Model file for the job. Use its own axes, mm. A direction names the side the tool comes from. Round coordinates to 2 decimals unless told otherwise and drop trailing zeros. Order: outer loops, then holes, each group sorted by start corner. A loop starts at its lowest first (then second) coordinate and runs counter-clockwise, first axis right, second up. Notation, with made-up numbers: (11.25, -25.75) - (68.25, -25.75) arc R18 cw to (68.25, -7.75) - close; hole circle Ø11 at (-5, 11.25). An arc over 180 degrees is marked (long way). Write item = value, one per line.
```python
from build123d import *

# Parameters (mm, degrees)
SKETCH_1_W          = 40
SKETCH_1_H          = 270
EXTRUDE_1_DEPTH     = 17
CUT_EXTRUDE_1_DEPTH = 6


with BuildPart() as part:
    # 스케치1 → 보스-돌출1 (new, symmetric)
    with BuildSketch(Plane(origin=(0, 0, 0), x_dir=(0, 0, -1), z_dir=(1, 0, 0))):
        with Locations((0, -135)):
            Rectangle(SKETCH_1_W, SKETCH_1_H)
    extrude(amount=EXTRUDE_1_DEPTH, both=True)

    # 스케치2 → 컷-돌출1 (cut, symmetric)
    with BuildSketch(Plane(origin=(0, 0, 0), x_dir=(0, 0, -1), z_dir=(1, 0, 0))):
        Polygon((-9.231313733, 0), (-9.231313733, -13.51839175), (-5.020847881, -120), (9.979152119, -120), (9.979152119, 0), align=None)
    extrude(amount=CUT_EXTRUDE_1_DEPTH, both=True, mode=Mode.SUBTRACT)


solid = part.part
```
1) Wall check: line 1 along X through (y, z) = (-89, 2); line 2 along Z through (x, y) = (-3, -64); line 3 along Z through (x, y) = (-3, -90). Give the ranges that are in metal, low to high.
Conclusion:
line_1 = -17 to -6, 6 to 17
line_2 = -20 to -9.98, 7.24 to 20
line_3 = -20 to -9.98, 6.21 to 20
2) 3-axis set-ups, long thin cutter, end or side, ignore diameter. For faces 1 (the face through (0, -7, 9.231)), 2 (the face through (0, -137, 20)): which of +Z, -Z, +X, -X, +Y, -Y reach the whole face in a straight line?
Conclusion:
face_1 = +Y
face_2 = +Z, +X, -X, +Y, -Y
3) Cut at D-D (y = -93.5). Write the cut outline in (x, z), and give its area (3 significant figures).
Conclusion:
outline = (-17, -20) - (17, -20) - (17, 20) - (-17, 20) - close; hole (-6, -9.98) - (6, -9.98) - (6, 6.07) - (-6, 6.07) - close
area = 1,170 mm^2
4) Mould opens along Z. For faces 3 (the face through (0, -137, -20)), 4 (the face through (0, -61, -9.979)), 5 (the face through (-17, -133, 0)) say: +Z half, -Z half, draft (parallel to the pull), parting line (faces both ways), or undercut.
Conclusion:
face_3 = -Z half
face_4 = undercut
face_5 = draft
5) Cut at A-A (z = 2.5). Write the cut outline in (x, y), and give its area (3 significant figures).
Conclusion:
outline = (-17, -270) - (17, -270) - (17, 0) - (6, 0) - (6, -120) - (-6, -120) - (-6, 0) - (-17, 0) - close
area = 7,740 mm^2
6) Cut at C-C (x = 2). Write the cut outline in (y, z), and give its area (3 significant figures).
Conclusion:
outline = (-270, -20) - (0, -20) - (0, -9.98) - (-120, -9.98) - (-120, 5.02) - (-13.52, 9.23) - (0, 9.23) - (0, 20) - (-270, 20) - close
area = 8,720 mm^2
7) Cut at B-B (y = -17.5). Write the cut outline in (x, z), and give its area (3 significant figures).
Conclusion:
outline = (-17, -20) - (17, -20) - (17, 20) - (-17, 20) - close; hole (-6, -9.98) - (6, -9.98) - (6, 9.07) - (-6, 9.07) - close
area = 1,130 mm^2
